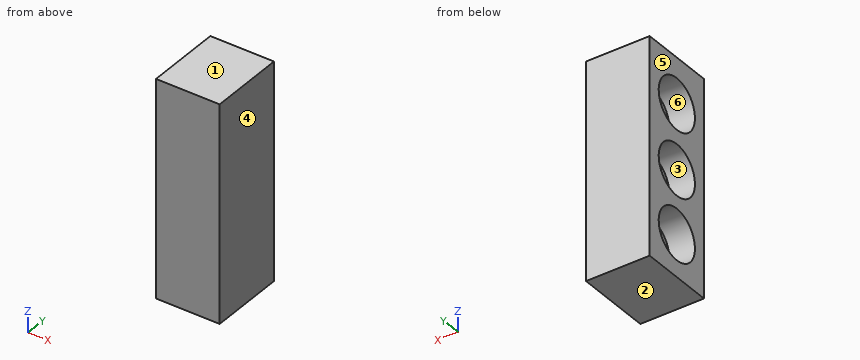
```python
from build123d import *

# Parameters (mm, degrees)
CYLINDER004_R          = 20
CYLINDER004_DEPTH      = 20
CYLINDER005_R          = 20
CYLINDER005_DEPTH      = 20
CYLINDER003_R          = 20
CYLINDER003_DEPTH      = 20
BOX009_W               = 170
BOX009_H               = 60
BOX009_DEPTH           = 50
CUT006_PLACEMENT_ANGLE = 90


with BuildPart() as cylinder003:
    # Cylinder004 → Cylinder004 (new body)
    with BuildSketch(Plane(origin=(83, 579, 175), x_dir=(1, 0, 0), z_dir=(0, 0, 1))):
        Circle(CYLINDER004_R)
    extrude(amount=CYLINDER004_DEPTH)


with BuildPart() as cylinder004:
    # Cylinder005 → Cylinder005 (new body)
    with BuildSketch(Plane(origin=(134, 579, 175), x_dir=(1, 0, 0), z_dir=(0, 0, 1))):
        Circle(CYLINDER005_R)
    extrude(amount=CYLINDER005_DEPTH)


with BuildPart() as cylinder002:
    # Cylinder003 → Cylinder003 (new body)
    with BuildSketch(Plane(origin=(33, 579, 175), x_dir=(1, 0, 0), z_dir=(0, 0, 1))):
        Circle(CYLINDER003_R)
    extrude(amount=CYLINDER003_DEPTH)


with BuildPart() as obj1:
    # Box009 → Box009 (new body)
    with BuildSketch(Plane(origin=(0, 549, 145), x_dir=(1, 0, 0), z_dir=(0, 0, 1))):
        with Locations((85, 30)):
            Rectangle(BOX009_W, BOX009_H)
    extrude(amount=BOX009_DEPTH)

    # Cut004: cut Cylinder002
    add(cylinder002.part, mode=Mode.SUBTRACT)

    # Cut005: cut Cylinder004
    add(cylinder004.part, mode=Mode.SUBTRACT)

    # Cut006: cut Cylinder003
    add(cylinder003.part, mode=Mode.SUBTRACT)


with BuildPart() as obj1_1:
    # Cut006 placement: moved
    add(obj1.part.moved(Location((363, -579, 130))).rotate(Axis((363, -579, 130), (0, -1, 0)), CUT006_PLACEMENT_ANGLE))


solid = obj1_1.part
```
Read the model definition and answer for the solid it produces. Units are mm, in the model's axes. Face numbers are marked on the shaded views. A direction names the side the tool comes from. Coordinates: 2 decimals unless noted, no trailing zeros. Write each loop counter-clockwise with the first axis right and the second up, starting at its lowest first coordinate (ties: lowest second). Pieces come first, ordered by that corner, then holes. Notation, with made-up numbers: (56.25, 38) - (110.25, 38) arc R7 ccw to (110.25, 45) - close; hole circle Ø3 at (11.25, 73.5). An arc over 180 degrees is marked (long way). Answer as a JSON object with one key per item and string values. Group by question number.
1. A cutting plane is placed at D-D (z = 147). Determine the outline of the cut face in (x, y).
2. A cutting plane is placed at A-A (x = 177.5). Determine the outline of the cut face in (y, z).
3. A cutting plane is placed at C-C (y = -9). Determine the outline of the cut face in (x, z).
4. Consider L1, parallel to Y at x = 175.75, z = 264; L2, parallel to Z at x = 177.5, y = 7 (3 decimals); L3, parallel to Z at x = 179.5, y = 6.5. Determine where each line is inside the solid, lowest interval first. Write a range as [from, to].
5. Which of the six approach directions +Z, -Z, +X, -X, +Y, -Y give full straight-line access (tool end or side, diameter ignored) to the marked faces 5 and 6?
6. A cutting plane is placed at B-B (z = 213). Determine the outline of the cut face in (x, y), plus the area to 3 significant figures.
7. This flat-tipped pin is pushed along its axis until it touches: P1, Ø20, axis at y = -7.5, z = 269.5, coming from the -X side. Where does it stop, or does it pass through?
8. The mould has two halves that part along Z. Classify the marked faces 1, 2, 3 and 4: +Z half, -Z half, draft (parallel to the pull), parting line (faces both ways), or undercut.
Worked out:
{
 "1": {"outline": "(168, -30) - (218, -30) - (218, 30) - (168, 30) - (168, 12) - (188, 12) - (188, -12) - (168, -12) - close"},
 "2": {"outline": "(-30, 130) - (30, 130) - (30, 300) - (-30, 300) - close; hole circle Ø40 at (0, 163); hole circle Ø40 at (0, 213); hole circle Ø40 at (0, 264)"},
 "3": {"outline": "(168, 130) - (218, 130) - (218, 300) - (168, 300) - (168, 281.86) - (188, 281.86) - (188, 246.14) - (168, 246.14) - (168, 230.86) - (188, 230.86) - (188, 195.14) - (168, 195.14) - (168, 180.86) - (188, 180.86) - (188, 145.14) - (168, 145.14) - close"},
 "4": {"L1": "y = [-30, -20], [20, 30]", "L2": "z = [130, 144.265], [181.735, 194.265], [231.735, 245.265], [282.735, 300]", "L3": "z = [130, 144.09], [181.91, 194.09], [231.91, 245.09], [282.91, 300]"},
 "5": {"face 5": "+Z, -Z, -X, +Y, -Y", "face 6": "-X"},
 "6": {"outline": "(168, -30) - (218, -30) - (218, 30) - (168, 30) - (168, 20) - (188, 20) - (188, -20) - (168, -20) - close", "area": "2,200 mm²"},
 "7": {"P1": "stops at x = 188"},
 "8": {"face 1": "+Z half", "face 2": "-Z half", "face 3": "undercut", "face 4": "draft"}
}
